```python
from build123d import *

# Parameters (mm, degrees)
ESQUISSE1_W                  = 52.5
ESQUISSE1_H                  = 57.5
ESQUISSE1_W_2                = 42.5
ESQUISSE1_H_2                = 47.5
EXTRU_MINCE1_DEPTH           = 20
ESQUISSE3_W                  = 6.75
ESQUISSE3_H                  = 41
ESQUISSE3_W_2                = 30.75
BOSS_EXTRU_1_DEPTH           = 52
ESQUISSE6_W                  = 5
ESQUISSE6_H                  = 23
ESQUISSE6_W_2                = 13.5
ESQUISSE6_H_2                = 5
BOSS_EXTRU_3_DEPTH           = 5
ENL_V_MAT_EXTRU_1_REACH      = 103.977
ESQUISSE2_R                  = 1.6
ENL_V_START                  = -3
ENL_V_MAT_EXTRU_2_DEPTH      = 3
ENL_V_MAT_EXTRU_3_DEPTH      = 119.640475808
ENL_V_MAT_EXTRU_4_DEPTH      = 99.458112921
ENL_V_MAT_EXTRU_5_DEPTH      = 89.991923791
ENL_V_MAT_EXTRU_5_DEPTH_BACK = 89.991923791
ESQUISSE10_W                 = 35.75
ESQUISSE10_H                 = 51
CHANFREIN1_SIZE2             = 4.195498156
CHANFREIN1_SIZE              = 5


with BuildPart() as part:
    # Esquisse1 → Extru.-Mince1 (new body)
    with BuildSketch(Plane(origin=(0, 0, 0), x_dir=(1, 0, 0), z_dir=(0, 1, 0))):
        Rectangle(ESQUISSE1_W, ESQUISSE1_H)
        Rectangle(ESQUISSE1_W_2, ESQUISSE1_H_2, mode=Mode.SUBTRACT)
    extrude(amount=EXTRU_MINCE1_DEPTH)

    # Esquisse3 → Boss.-Extru.1 (add)
    with BuildSketch(Plane.XZ):
        Polygon((26.25, 28.75), (38, 28.75), (38, -22.25), (21.25, -22.25), (21.25, 23.75), (-21.25, 23.75), (-21.25, -22.25), (-62, -22.25), (-62, 28.75), (-26.25, 28.75), (0, 28.75), align=None)
        with Locations((29.625, 3.25)):
            Rectangle(ESQUISSE3_W, ESQUISSE3_H, mode=Mode.SUBTRACT)
        with Locations((-41.625, 3.25)):
            Rectangle(ESQUISSE3_W_2, ESQUISSE3_H, mode=Mode.SUBTRACT)
    extrude(amount=-BOSS_EXTRU_1_DEPTH)

    # Esquisse6 → Boss.-Extru.3 (add)
    with BuildSketch(Plane(origin=(0, 52, 0), x_dir=(1, 0, 0), z_dir=(0, 1, 0))):
        with Locations((35.5, -5.25)):
            Rectangle(ESQUISSE6_W, ESQUISSE6_H)
        with Locations((16.25, -26.25)):
            Rectangle(ESQUISSE6_W_2, ESQUISSE6_H_2)
        with Locations((-12.25, -26.25)):
            Rectangle(ESQUISSE6_W_2, ESQUISSE6_H_2)
        with Locations((-40.75, -26.25)):
            Rectangle(ESQUISSE6_W_2, ESQUISSE6_H_2)
        with Locations((-40.75, 19.75)):
            Rectangle(ESQUISSE6_W_2, ESQUISSE6_H_2)
        with Locations((-59.5, -5.25)):
            Rectangle(ESQUISSE6_W, ESQUISSE6_H)
    boss_extru_3 = extrude(amount=BOSS_EXTRU_3_DEPTH)

    # Esquisse2 → Enlèv. mat.-Extru.1 (cut, up to next)
    with BuildSketch(Plane.XY.offset(28.75), mode=Mode.PRIVATE) as enl_v_mat_extru_1_sk1:
        with Locations((-15.5, 5.2)):
            Circle(ESQUISSE2_R)
    enl_v_mat_extru_1_tool1 = extrude(enl_v_mat_extru_1_sk1.sketch, amount=-ENL_V_MAT_EXTRU_1_REACH, mode=Mode.PRIVATE) & part.part
    # Esquisse2 → Enlèv. mat.-Extru.1 (cut, up to next)
    with BuildSketch(Plane.XY.offset(28.75), mode=Mode.PRIVATE) as enl_v_mat_extru_1_sk2:
        with Locations((15.5, 5.2)):
            Circle(ESQUISSE2_R)
    enl_v_mat_extru_1_tool2 = extrude(enl_v_mat_extru_1_sk2.sketch, amount=-ENL_V_MAT_EXTRU_1_REACH, mode=Mode.PRIVATE) & part.part
    # Esquisse2 → Enlèv. mat.-Extru.1 (cut, up to next)
    with BuildSketch(Plane.XY.offset(28.75), mode=Mode.PRIVATE) as enl_v_mat_extru_1_sk3:
        with Locations(Location((15.5, 34.8, 0), (0, 0, 180))):
            Circle(ESQUISSE2_R)
    enl_v_mat_extru_1_tool3 = extrude(enl_v_mat_extru_1_sk3.sketch, amount=-ENL_V_MAT_EXTRU_1_REACH, mode=Mode.PRIVATE) & part.part
    # Esquisse2 → Enlèv. mat.-Extru.1 (cut, up to next)
    with BuildSketch(Plane.XY.offset(28.75), mode=Mode.PRIVATE) as enl_v_mat_extru_1_sk4:
        with Locations(Location((-15.5, 34.8, 0), (0, 0, 180))):
            Circle(ESQUISSE2_R)
    enl_v_mat_extru_1_tool4 = extrude(enl_v_mat_extru_1_sk4.sketch, amount=-ENL_V_MAT_EXTRU_1_REACH, mode=Mode.PRIVATE) & part.part
    # Esquisse2 → Enlèv. mat.-Extru.1 (cut, up to next)
    with BuildSketch(Plane.XY.offset(28.75), mode=Mode.PRIVATE) as enl_v_mat_extru_1_sk5:
        with BuildLine():
            Line((2.65, 36.215870824), (2.65, 32.215870824))
            ThreePointArc((2.65, 32.215870824), (0, 7.5), (-2.65, 32.215870824))
            Line((-2.65, 32.215870824), (-2.65, 36.215870824))
            ThreePointArc((-2.65, 36.215870824), (0, 38.865870824), (2.65, 36.215870824))
        make_face()
    enl_v_mat_extru_1_tool5 = extrude(enl_v_mat_extru_1_sk5.sketch, amount=-ENL_V_MAT_EXTRU_1_REACH, mode=Mode.PRIVATE) & part.part
    add(enl_v_mat_extru_1_tool1.solids().sort_by_distance((-15.5, 5.2, 28.75))[0], mode=Mode.SUBTRACT)
    add(enl_v_mat_extru_1_tool2.solids().sort_by_distance((15.5, 5.2, 28.75))[0], mode=Mode.SUBTRACT)
    add(enl_v_mat_extru_1_tool3.solids().sort_by_distance((15.5, 34.8, 28.75))[0], mode=Mode.SUBTRACT)
    add(enl_v_mat_extru_1_tool4.solids().sort_by_distance((-15.5, 34.8, 28.75))[0], mode=Mode.SUBTRACT)
    add(enl_v_mat_extru_1_tool5.solids().sort_by_distance((0, 20.91985, 28.75))[0], mode=Mode.SUBTRACT)

    # Esquisse4 → Enlèv. mat.-Extru.2 (cut)
    with BuildSketch(Plane(origin=(0, 0, 23.75), x_dir=(-1, 0, 0), z_dir=(0, 0, -1)).offset(ENL_V_START)):
        with BuildLine():
            Line((-12.5, 20), (-12.5, 57))
            Line((-12.5, 57), (12.5, 57))
            Line((12.5, 57), (12.5, 20))
            ThreePointArc((12.5, 20), (0, 32.5), (-12.5, 20))
        make_face()
    extrude(amount=ENL_V_MAT_EXTRU_2_DEPTH, mode=Mode.SUBTRACT)

    # Symétrie1: Boss.-Extru.3 across plane
    add(boss_extru_3.mirror(Plane(origin=(0, 26, 0), x_dir=(0, 0, 1), z_dir=(0, -1, 0))))

    # Esquisse7 → Enlèv. mat.-Extru.3 (cut, through all)
    with BuildSketch(Plane(origin=(38, 0, 0), x_dir=(0, 0, -1), z_dir=(1, 0, 0))):
        with BuildLine():
            Line((-11.75, 45), (5.25, 45))
            ThreePointArc((5.25, 45), (12.321067812, 42.071067812), (15.25, 35))
            Line((15.25, 35), (15.25, 17))
            ThreePointArc((15.25, 17), (12.321067812, 9.928932188), (5.25, 7))
            Line((5.25, 7), (-11.75, 7))
            ThreePointArc((-11.75, 7), (-18.821067812, 9.928932188), (-21.75, 17))
            Line((-21.75, 17), (-21.75, 35))
            ThreePointArc((-21.75, 35), (-18.821067812, 42.071067812), (-11.75, 45))
        make_face()
    extrude(amount=-ENL_V_MAT_EXTRU_3_DEPTH, mode=Mode.SUBTRACT)

    # Esquisse8 → Enlèv. mat.-Extru.4 (cut, through all)
    with BuildSketch(Plane(origin=(0, 0, -22.25), x_dir=(-1, 0, 0), z_dir=(0, 0, -1))):
        with BuildLine():
            Line((48.625, 33.5), (48.625, 18.5))
            ThreePointArc((48.625, 18.5), (41.625, 11.5), (34.625, 18.5))
            Line((34.625, 18.5), (34.625, 33.5))
            ThreePointArc((34.625, 33.5), (41.625, 40.5), (48.625, 33.5))
        make_face()
    extrude(amount=-ENL_V_MAT_EXTRU_4_DEPTH, mode=Mode.SUBTRACT)

    # Esquisse10 → Enlèv. mat.-Extru.5 (cut, two sides: drawn at the far end of the back side and taken through both)
    with BuildSketch(Plane(origin=(0, 52, 0), x_dir=(1, 0, 0), z_dir=(0, 1, 0)).offset(-ENL_V_MAT_EXTRU_5_DEPTH_BACK)):
        with Locations((-44.125, -3.25)):
            Rectangle(ESQUISSE10_W, ESQUISSE10_H)
    extrude(amount=ENL_V_MAT_EXTRU_5_DEPTH + ENL_V_MAT_EXTRU_5_DEPTH_BACK, mode=Mode.SUBTRACT)

    # Chanfrein1
    chanfrein1_edges = [part.edges().sort_by_distance(p)[0] for p in [
        (0, 20, -23.75),
    ]]
    chanfrein1_side = [part.faces().sort_by_distance(p)[0] for p in [
        (0, 20, -23.833909963),
    ]]
    chamfer(chanfrein1_edges, length=CHANFREIN1_SIZE - 0.0001, length2=CHANFREIN1_SIZE2 - 0.0001, reference=chanfrein1_side[0])  # a hair under: the kernel refuses the full size


solid = part.part
```
Source: CAD feature listing. Evaluate the final solid. Frame: model axes, mm. A direction names the side the tool comes from. Round coordinates to 2 decimals unless told otherwise and drop trailing zeros. Loops run counter-clockwise (first coordinate to the right, second up) from the corner with the lowest first, then second, coordinate; pieces in that order, holes last. Notation, with made-up numbers: M 67,73 L 106,73 A33 ccw 106,109 Z; hole C -23.75,33 d7. An arc over 180 degrees is marked long. Put each result on its own line as item: value.
(1) Section C-C, the plane y = 5.2. Return loops of the section in (x, z).
Solutions:
outline: M -26.25,-28.75 L 26.25,-28.75 L 26.25,-22.25 L 38,-22.25 L 38,28.75 L 17.1,28.75 L 17.1,23.75 L 21.25,23.75 L 21.25,-23.75 L -21.25,-23.75 L -21.25,23.75 L -17.1,23.75 L -17.1,28.75 L -26.25,28.75 Z; M -13.9,23.75 L 13.9,23.75 L 13.9,28.75 L -13.9,28.75 Z; hole M 26.25,-17.25 L 33,-17.25 L 33,23.75 L 26.25,23.75 Z
(2) Ray query, line 1 (X direction, y = 34.8, z = 27.2); line 2 (X direction, y = 17, z = -16.5); line 3 (Y direction, x = -15.5, z = 26.45). Return the intervals inside material, ascending. Write a range as [from, to].
Solutions:
line 1: [-26.25, -17.1], [-13.9, -2.65], [2.65, 13.9], [17.1, 38]
line 2: [-26.25, -21.25], [21.25, 26.25], [33, 38]
line 3: [-5, 3.6], [6.8, 33.2], [36.4, 57]
(3) Pull-direction query (Z, two-part tool) for faces 1 (the face through (-26.25, 26, -19)), 2 (the face through (35, -2, 16.75)), 3 (the face through (24, 7, 3)); classes: released by +Z, released by -Z, zero draft, split by the parting line, or undercut.
Solutions:
face 1: zero draft
face 2: released by +Z
face 3: undercut
(4) Section D-D, the plane x = 28. Return loops of the section in (y, z).
Solutions:
outline: M 0,-22.25 L 52,-22.25 L 52,-17.25 L 0,-17.25 Z; M 0,23.75 L 52,23.75 L 52,28.75 L 0,28.75 Z
(5) Section B-B, the plane z = 3. Return loops of the section in (x, y).
Solutions:
outline: M -26.25,0 L -21.25,0 L -21.25,7 L -26.25,7 Z; M -26.25,45 L -21.25,45 L -21.25,52 L -26.25,52 Z; M 21.25,0 L 26.25,0 L 26.25,7 L 21.25,7 Z; M 21.25,45 L 26.25,45 L 26.25,52 L 21.25,52 Z; M 33,-5 L 38,-5 L 38,7 L 33,7 Z; M 33,45 L 38,45 L 38,57 L 33,57 Z
(6) Access query for faces 4 (the face through (13.9, 5.27, 26.28)), 5 (the face through (35.53, 41.99, 18.9)), 6 (the face through (23, 54, 26)), 7 (the face through (2.65, 34, 28)), 8 (the face through (26.25, 6.6, 3.2)). Directions: +Z, -Z, +X, -X, +Y, -Y. A direction counts if a zero-diameter tool reaches every point of the face in a straight line with its end or side. Return the directions, or none.
Solutions:
face 4: +Z
face 5: +X, -X
face 6: +Z, -Z, +X, +Y
face 7: +Z, -Z
face 8: +Y, -Y
(7) First-contact query: pin 1 (4 mm diameter, centred on x = 23.5, z = 2.5, fed in from +Y); pin 2 (2.5 mm diameter, centred on y = -3, z = 27, fed in from -X); pin 3 (1.5 mm diameter, centred on x = -24.5, y = 29, fed in from -Z); pin 4 (2 mm diameter, centred on x = 19, z = 20, fed in from +Y). Flat tips, straight axial feed; report the tip coordinate or a pass-through.
Solutions:
pin 1: y = 52
pin 2: x = -19
pin 3: z = -22.25
pin 4: through
(8) Section A-A, the plane x = 0. State how many separate pieces and enclosed holes the cut face has, and give its area (3 significant figures).
Solutions:
separate pieces: 3
enclosed holes: 0
area: 153 mm²
